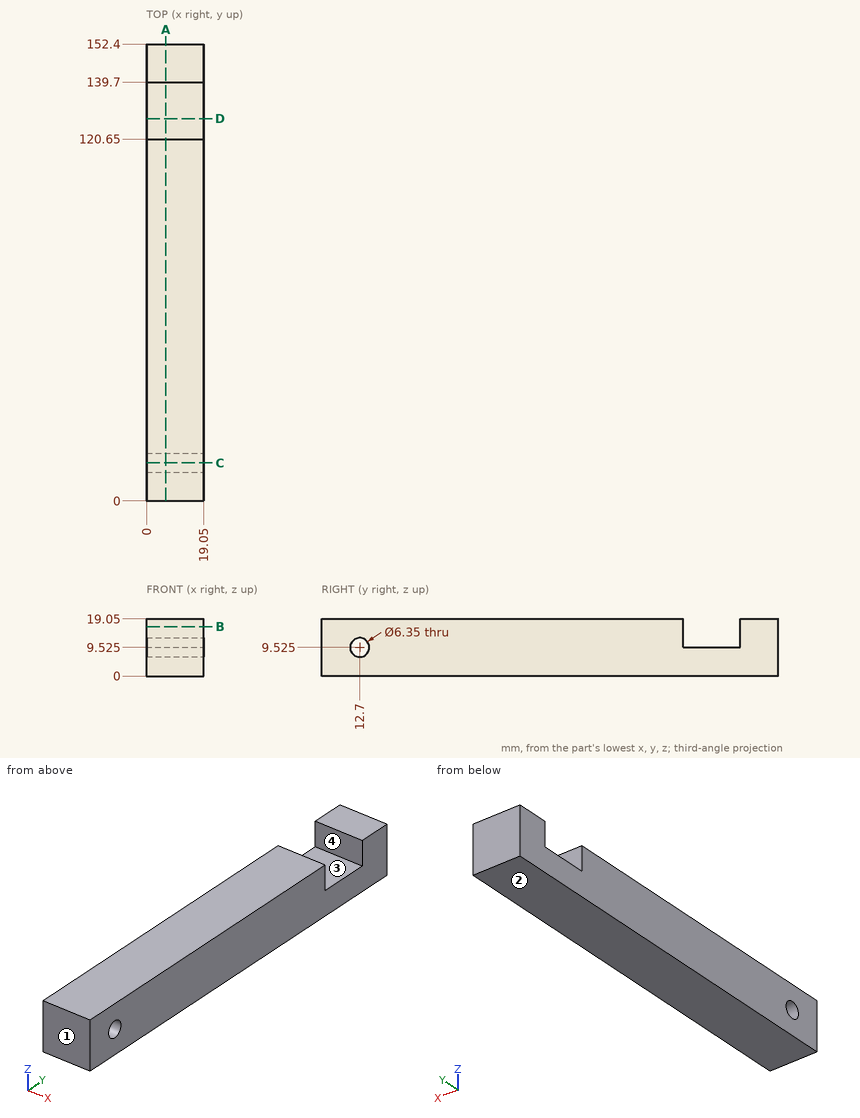
Can you work these out from the drawing? Everything is in mm from the part's minimum corner. Give positions to 0.01 mm unless a question says otherwise; leave off trailing zeros. Order: outer loops, then holes, each group sorted by start corner. A loop starts at its lowest first (then second) coordinate and runs counter-clockwise, first axis right, second up. Notation, with made-up numbers: (42, 53) -> (83, 53) arc R19 ccw to (83, 78) -> close; hole circle Ø7 at (-37.75, 9). An arc over 180 degrees is marked (long way). Return JSON: item names as keys, results as strings.
1. Imagine slicing it at A-A on x = 6.5. List the corners of the cut face in (y, z) for me (3 decimals), then the cut area to 3 significant figures.
Answer list:
{"outline": "(0, 0) -> (152.4, 0) -> (152.4, 19.05) -> (139.7, 19.05) -> (139.7, 9.525) -> (120.65, 9.525) -> (120.65, 19.05) -> (0, 19.05) -> close; hole circle Ø6.35 at (12.7, 9.525)", "area": "2,690 mm2"}
2. For pin 1 Ø9.5 at (x, y) = (7.5, 128) entering from +Z (3 decimals), with a flat end and sliding along its axis, tell me the tip position at first contact or that it passes through.
Answer list:
{"pin 1": "stops at z = 9.525"}
3. Imagine slicing it at C-C on y = 12.7. List the corners of the cut face in (x, z) for me, then the cut area to 3 significant figures.
Answer list:
{"outline": "(0, 0) -> (19.05, 0) -> (19.05, 6.35) -> (0, 6.35) -> close; (0, 12.7) -> (19.05, 12.7) -> (19.05, 19.05) -> (0, 19.05) -> close", "area": "242 mm2"}
4. I need wall thicknesses on line 1 (Z direction, x = 7.25, y = 12.7); line 2 (Y direction, x = 12, z = 14.5); line 3 (Z direction, x = 4.5, y = 131.5) (3 decimals). Which ranges of each line are inside material? Lowest first, please. Write a range as from..to.
Answer list:
{"line 1": "z = 0..6.35, 12.7..19.05", "line 2": "y = 0..120.65, 139.7..152.4", "line 3": "z = 0..9.525"}
5. Imagine slicing it at D-D on y = 127.5. List the corners of the cut face in (x, z) for me (3 decimals).
Answer list:
{"outline": "(0, 0) -> (19.05, 0) -> (19.05, 9.525) -> (0, 9.525) -> close"}
6. Imagine slicing it at B-B on z = 16.5. List the corners of the cut face in (x, y) for me.
Answer list:
{"outline": "(0, 0) -> (19.05, 0) -> (19.05, 120.65) -> (0, 120.65) -> close; (0, 139.7) -> (19.05, 139.7) -> (19.05, 152.4) -> (0, 152.4) -> close"}
7. Thinking about a two-plate mould opening in Y: for the marked faces 1, 2, 3 and 4, which applies, pulls with the +Y half, pulls with the -Y half, needs draft (parallel to the pull), parting line crosses it, or undercut?
Answer list:
{"face 1": "pulls with the -Y half", "face 2": "needs draft", "face 3": "undercut", "face 4": "undercut"}
